Geometry check sheet. Reference: the model listing, model coordinates, mm. Give positions to 0.01 mm unless a question says otherwise; leave off trailing zeros. Loops run counter-clockwise (first coordinate to the right, second up) from the corner with the lowest first, then second, coordinate; pieces in that order, holes last. Notation, with made-up numbers: (59.5, -30.75) - (110.5, -30.75) arc R16 ccw to (110.5, -1.75) - close; hole circle Ø11 at (-1, 80.25). An arc over 180 degrees is marked (long way). Use a Markdown table: item, result. Add a question column.
1. Draft check along X on faces 1 (the cylindrical face through (38.5, 3, -0.2)), 2 (the flat face through (20, 9, 0)). Enter one of: pulls with the +X half, pulls with the -X half, needs draft (parallel to the pull), parting line crosses it, or undercut.
2. Material ranges on L1, parallel to Y at x = 7, z = -0.2; L2, parallel to Y at x = 12.88, z = -0.2; L3, parallel to Y at x = 17, z = -0.15, recorded low to high.
3. Cross-section at D-D on z = -0.2. Count the separate pieces of the cut face and the enclosed holes in it, and give its area (3 significant figures).
4. Cross-section at B-B on y = 16. Enter the section's corners in (x, z), and give its area (3 significant figures).
5. Cross-section at C-C on x = 23.04. Enter the section's corners in (y, z), and give its area (3 significant figures).
6. Cross-section at A-A on x = 38. Enter the section's corners in (y, z).
from build123d import *

# Parameters (mm, degrees)
SKETCH_1_R      = 0.499999
SKETCH_1_W      = 24.49999926
SKETCH_1_H      = 11.00000086
EXTRUDE_1_DEPTH = 0.41148


with BuildPart() as part:
    # 草图1 → 凸台-拉伸1 (new body)
    with BuildSketch(Plane.XY):
        Polygon((1.5257399, 2.2389465), (1.6265017, 1.99568562), (1.78679094, 1.78679094), (1.99568562, 1.6265017), (2.2389465, 1.5257399), (2.50000008, 1.49137116), (38.4999992, 1.49999954), (38.4999992, 1.49137116), (38.76105278, 1.5257399), (39.00431366, 1.6265017), (39.21320834, 1.78679094), (39.37349758, 1.99568562), (39.47425938, 2.2389465), (39.50862812, 2.50000008), (39.49999974, 28.49999888), (39.50862812, 28.49999888), (39.47425938, 28.76105246), (39.37349758, 29.00431334), (39.21320834, 29.21320802), (39.00431366, 29.37349726), (38.76105278, 29.47425906), (38.4999992, 29.5086278), (2.50000008, 29.49999942), (2.50000008, 29.5086278), (2.2389465, 29.47425906), (1.99568562, 29.37349726), (1.78679094, 29.21320802), (1.6265017, 29.00431334), (1.5257399, 28.76105246), (1.49137116, 28.49999888), (1.49999954, 2.50000008), (1.49137116, 2.50000008), align=None)
        with Locations(Location((38.0000002, 28.00000242, 0), (0, 0, 180))):
            Circle(SKETCH_1_R, mode=Mode.SUBTRACT)
        with Locations(Location((34.00000058, 24.00000026, 0), (0, 0, 180))):
            Circle(SKETCH_1_R, mode=Mode.SUBTRACT)
        with Locations(Location((30.65999964, 23.24999922, 0), (0, 0, 180))):
            Circle(SKETCH_1_R, mode=Mode.SUBTRACT)
        with Locations(Location((28.11999964, 23.24999922, 0), (0, 0, 180))):
            Circle(SKETCH_1_R, mode=Mode.SUBTRACT)
        with Locations(Location((23.03999964, 23.24999922, 0), (0, 0, 180))):
            Circle(SKETCH_1_R, mode=Mode.SUBTRACT)
        with Locations(Location((20.49999964, 23.24999922, 0), (0, 0, 180))):
            Circle(SKETCH_1_R, mode=Mode.SUBTRACT)
        with Locations(Location((25.57999964, 23.24999922, 0), (0, 0, 180))):
            Circle(SKETCH_1_R, mode=Mode.SUBTRACT)
        with Locations(Location((30.65999964, 7.74999974, 0), (0, 0, 180))):
            Circle(SKETCH_1_R, mode=Mode.SUBTRACT)
        with Locations(Location((28.11999964, 7.74999974, 0), (0, 0, 180))):
            Circle(SKETCH_1_R, mode=Mode.SUBTRACT)
        with Locations(Location((38.0000002, 3.00000162, 0), (0, 0, 180))):
            Circle(SKETCH_1_R, mode=Mode.SUBTRACT)
        with Locations(Location((34.00000058, 7.00000124, 0), (0, 0, 180))):
            Circle(SKETCH_1_R, mode=Mode.SUBTRACT)
        with Locations(Location((23.03999964, 7.74999974, 0), (0, 0, 180))):
            Circle(SKETCH_1_R, mode=Mode.SUBTRACT)
        with Locations(Location((20.49999964, 7.74999974, 0), (0, 0, 180))):
            Circle(SKETCH_1_R, mode=Mode.SUBTRACT)
        with Locations(Location((25.57999964, 7.74999974, 0), (0, 0, 180))):
            Circle(SKETCH_1_R, mode=Mode.SUBTRACT)
        with Locations(Location((15.41999964, 23.24999922, 0), (0, 0, 180))):
            Circle(SKETCH_1_R, mode=Mode.SUBTRACT)
        with Locations(Location((12.87999964, 23.24999922, 0), (0, 0, 180))):
            Circle(SKETCH_1_R, mode=Mode.SUBTRACT)
        with Locations(Location((17.95999964, 23.24999922, 0), (0, 0, 180))):
            Circle(SKETCH_1_R, mode=Mode.SUBTRACT)
        with Locations(Location((7.00000124, 24.00000026, 0), (0, 0, 180))):
            Circle(SKETCH_1_R, mode=Mode.SUBTRACT)
        with Locations(Location((2.99999908, 28.00000242, 0), (0, 0, 180))):
            Circle(SKETCH_1_R, mode=Mode.SUBTRACT)
        with Locations(Location((10.33999964, 23.24999922, 0), (0, 0, 180))):
            Circle(SKETCH_1_R, mode=Mode.SUBTRACT)
        with Locations(Location((15.41999964, 7.74999974, 0), (0, 0, 180))):
            Circle(SKETCH_1_R, mode=Mode.SUBTRACT)
        with Locations(Location((12.87999964, 7.74999974, 0), (0, 0, 180))):
            Circle(SKETCH_1_R, mode=Mode.SUBTRACT)
        with Locations(Location((17.95999964, 7.74999974, 0), (0, 0, 180))):
            Circle(SKETCH_1_R, mode=Mode.SUBTRACT)
        with Locations(Location((10.33999964, 7.74999974, 0), (0, 0, 180))):
            Circle(SKETCH_1_R, mode=Mode.SUBTRACT)
        with Locations(Location((7.00000124, 7.00000124, 0), (0, 0, 180))):
            Circle(SKETCH_1_R, mode=Mode.SUBTRACT)
        with Locations(Location((2.99999908, 3.00000162, 0), (0, 0, 180))):
            Circle(SKETCH_1_R, mode=Mode.SUBTRACT)
        with Locations((21.24999941, 15.50000075)):
            Rectangle(SKETCH_1_W, SKETCH_1_H, mode=Mode.SUBTRACT)
    extrude(amount=-EXTRUDE_1_DEPTH)


solid = part.part
Values found:
| question | item | result |
|---|---|---|
| 1 | face 1 | undercut |
| 1 | face 2 | needs draft |
| 2 | L1 | y = 1.49 to 6.5, 7.5 to 23.5, 24.5 to 29.5 |
| 2 | L2 | y = 1.49 to 7.25, 8.25 to 10, 21 to 22.75, 23.75 to 29.5 |
| 2 | L3 | y = 1.49 to 10, 21 to 29.5 |
| 3 | separate pieces | 1 |
| 3 | enclosed holes | 27 |
| 3 | area | 774 mm2 |
| 4 | outline | (1.5, -0.41) - (9, -0.41) - (9, 0) - (1.5, 0) - close; (33.5, -0.41) - (39.5, -0.41) - (39.5, 0) - (33.5, 0) - close |
| 4 | area | 5.56 mm2 |
| 5 | outline | (1.5, -0.41) - (7.25, -0.41) - (7.25, 0) - (1.5, 0) - close; (8.25, -0.41) - (10, -0.41) - (10, 0) - (8.25, 0) - close; (21, -0.41) - (22.75, -0.41) - (22.75, 0) - (21, 0) - close; (23.75, -0.41) - (29.5, -0.41) - (29.5, 0) - (23.75, 0) - close |
| 5 | area | 6.18 mm2 |
| 6 | outline | (1.5, -0.41) - (2.5, -0.41) - (2.5, 0) - (1.5, 0) - close; (3.5, -0.41) - (27.5, -0.41) - (27.5, 0) - (3.5, 0) - close; (28.5, -0.41) - (29.51, -0.41) - (29.51, 0) - (28.5, 0) - close |
